Print and shaded views of the part. All mm, measured from the part's lowest x, y and z. A direction names the side the tool comes from. Coordinates: 2 decimals unless noted, no trailing zeros. Order: outer loops, then holes, each group sorted by start corner. A loop starts at its lowest first (then second) coordinate and runs counter-clockwise, first axis right, second up. Notation, with made-up numbers: (-5.75, 46.25) -> (21.25, 46.25) arc R11 ccw to (21.25, 50.25) -> close; hole circle Ø8 at (52, -15.5). An arc over 180 degrees is marked (long way). Write item = value, one per line. Start each with the question number.
Q1. Cut at C-C, the plane z = 4.5. List the corners of the cut face in (x, y) (1 decimal).
Q2. 3-axis set-ups, long thin cutter, end or side, ignore diameter. For the marked faces 1, 2, 3, 4 and 5: which of +Z, -Z, +X, -X, +Y, -Y reach the whole face in a straight line?
Q3. Cut at A-A, the plane y = 3.5. List the corners of the cut face in (x, z).
Q4. Cut at B-B, the plane x = 5.75. List the corners of the cut face in (y, z) (1 decimal).
Q5. Mould opens along Y. For the marked faces 6, 7 and 8 say: +Y half, -Y half, draft (parallel to the pull), parting line (faces both ways), or undercut.
Q6. Cut at D-D, the plane x = 9.5. List the corners of the cut face in (y, z), plus the area to 3 significant figures.
Q7. Wall check: line 1 (Z direction, x = 7.25, y = 11.25); line 2 (X direction, y = 7.5, z = 5.25); line 3 (X direction, y = 6.25, z = 4.5). Give the ranges that are in metal, low to high. Write a range as from..to.
Q8. Flat gauge pins, fed straight in: pin 1 (1.5 mm diameter, centred on x = 6.5, z = 1, fed in from +Y) (3 decimals); pin 2 (2 mm diameter, centred on x = 5.5, z = 0.5, fed in from -Y) (3 decimals). Where does each tip first touch, or does it go through?
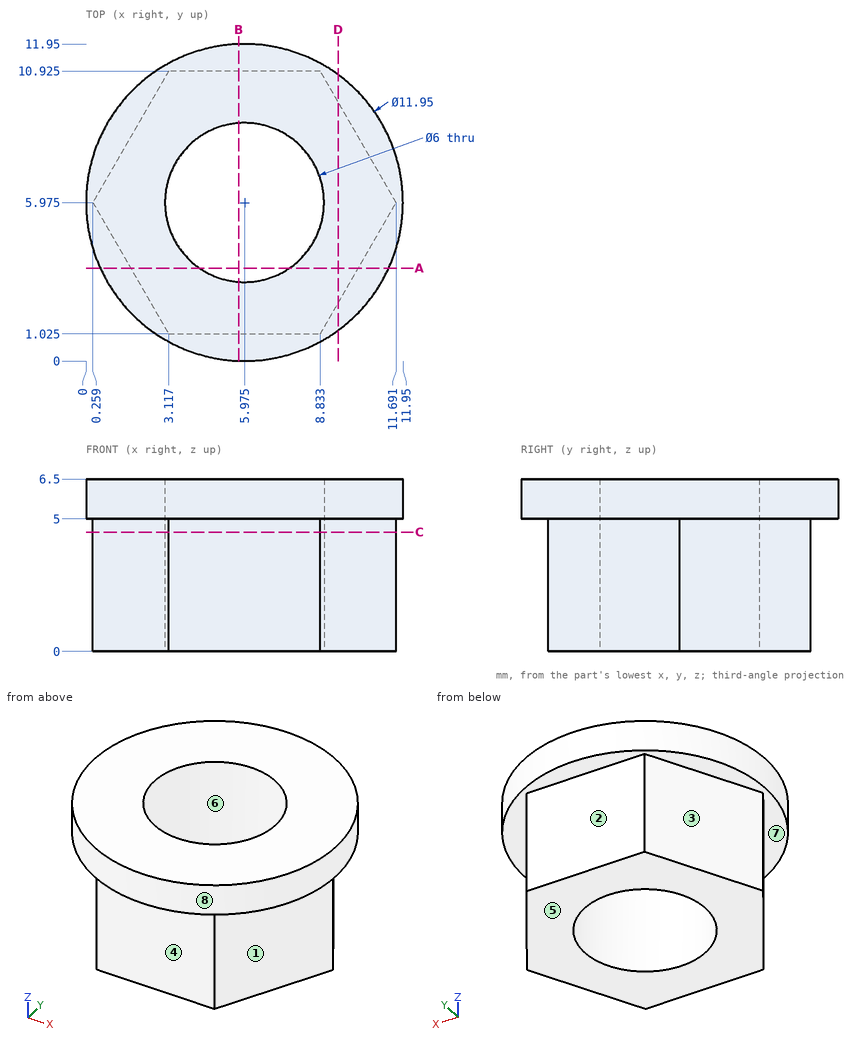
Here are the results:
q1.outline = (0.3, 6) -> (3.1, 1) -> (8.8, 1) -> (11.7, 6) -> (8.8, 10.9) -> (3.1, 10.9) -> close; hole circle Ø6 at (6, 6)
q2.face_1 = -Z, +X, -Y
q2.face_2 = -Z, +X, -X, +Y
q2.face_3 = -Z, -X, +Y
q2.face_4 = -Z, +X, -X, -Y
q2.face_5 = -Z, +X, -X, +Y, -Y
q3.outline = (0.54, 5) -> (1.69, 5) -> (1.69, 0) -> (4.28, 0) -> (4.28, 6.5) -> (0.54, 6.5) -> close; (7.67, 0) -> (10.26, 0) -> (10.26, 5) -> (11.41, 5) -> (11.41, 6.5) -> (7.67, 6.5) -> close
q4.outline = (0, 5) -> (1, 5) -> (1, 0) -> (3, 0) -> (3, 6.5) -> (0, 6.5) -> close; (9, 0) -> (10.9, 0) -> (10.9, 5) -> (11.9, 5) -> (11.9, 6.5) -> (9, 6.5) -> close
q5.face_6 = undercut
q5.face_7 = draft
q5.face_8 = parting line
q6.outline = (1.15, 5) -> (2.18, 5) -> (2.18, 0) -> (9.77, 0) -> (9.77, 5) -> (10.8, 5) -> (10.8, 6.5) -> (1.15, 6.5) -> close
q6.area = 52.4 mm²
q7.line_1 = 5..6.5
q7.line_2 = 0.2..3.39, 8.56..11.75
q7.line_3 = 0.42..2.99, 8.96..11.53
q8.pin_1 = 10.925
q8.pin_2 = 1.025
